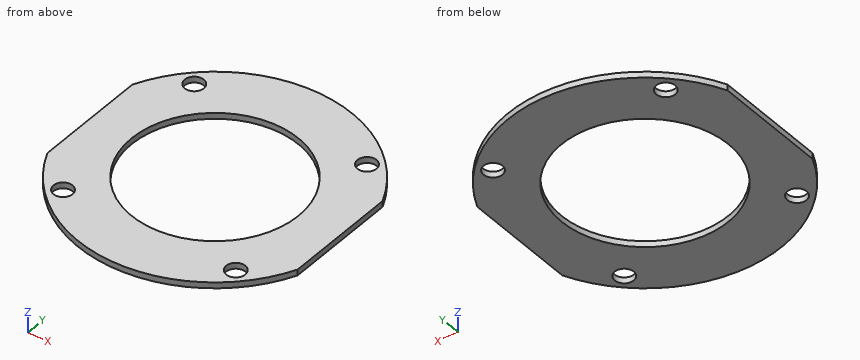
Autodesk Inventor part; units mm, degrees
ref_plane "Work Plane1" through (22, -12.0416, 0) normal (1, 0, 0) x (0, 0, -1)
ref_plane "YZ Plane" through (0, 0, 0) normal (1, 0, 0) x (0, 1, 0)
ref_plane "XZ Plane" through (0, 0, 0) normal (0, 1, 0) x (-1, 0, 0)
sketch "Sketch1" plane through (0, 0, 0) normal (0, 0, 1) x (1, 0, 0)
  circle A0 centre (0, 0) radius 14
  circle A1 centre (0, 0) radius 23
  dimension "d0" = 28
  dimension "d1" = 46
extrude "Extrusion1" add sketch "Sketch1" along normal blind 10
sketch "Sketch2" plane through (0, 0, 10) normal (0, 0, 1) x (1, 0, 0)
  line L0 (0, 0) -> (23, 0) construction
  circle A0 centre (0, 0) radius 23
  circle A1 centre (0, 0) radius 20.5 construction
  line L1 (0, 0) -> (14.4957, 14.4957) construction
  dimension "d35" = 41
  dimension "d34" = 45
hole "For-m3-screws" at (14.4957, 14.4957, 10) direction (0, 0, -1) diameter 3.2 end through all counterbore diameter 7 counterbore depth 8.5
fillet "Fillet3" radius 0.5 2 edges at (14.3283, 17.9917, 5.75) (17.9917, 14.3283, 5.75)
pattern_circular "Circular Pattern1" count 4 over 360 about axis through (0, 0, 0) along (0, 0, 1) of "For-m3-screws", "Fillet3"
sketch "Sketch3" plane through (0, 0, 0) normal (0, 1, 0) x (-1, 0, 0)
  line L0 (23, 3.8135) -> (-23, 1)
  line L1 (-23, 1) -> (-23, 11)
  line L2 (23, 10) -> (-27, 10)
  line L3 (-23, 11) -> (23, 11)
  line L4 (23, 11) -> (23, 3.8135)
  line L5 (-23, 0) -> (-23, 10)
  line L6 (23, 0) -> (23, 10)
  line L7 (-14, 0) -> (14, 0)
  line L8 (-27, 10) -> (-23, 10)
  point P0 (0, 0)
  point P1 (-14.3283, 10)
  point P2 (0, 11)
  point P3 (-17.9917, 10)
  dimension "d14" = 3.5
  dimension "d15" = 1
  dimension "d16" = 1
extrude "Angled-cut" [suppressed]
sketch "Sketch6" plane through (0, 0, 0) normal (0, 1, 0) x (-1, 0, 0)
  line L0 (23, 10) -> (-23, 10)
  line L1 (-23, 10) -> (-23, 1)
  line L2 (-23, 1) -> (23, 1)
  line L3 (23, 1) -> (23, 10)
  line L4 (23, 0) -> (-23, 0)
  line L5 (23, 0) -> (23, 10)
  line L6 (-23, 0) -> (-23, 10)
  point P0 (0, 0)
  point P1 (0, 10)
  dimension "d27" = 1
extrude "Straight-cut" cut sketch "Sketch6" along normal through all both and the other way through all contours L3 L2 L1 L0
sketch "Sketch4" plane through (0, 0, 0) normal (0, 0, 1) x (1, 0, 0)
  line L0 (21, 30) -> (26, 30)
  line L1 (26, 30) -> (26, -30)
  line L2 (26, -30) -> (21, -30)
  line L3 (21, -30) -> (21, 30)
  point P0 (0, 0)
  point P1 (26, 0)
  dimension "d19" = 21
  dimension "d20" = 60
  dimension "d21" = 5
extrude "Extrusion3" cut sketch "Sketch4" along normal blind 10
mirror "Mirror1" about plane through (0, 0, 0) normal (1, 0, 0) of "Extrusion3"
ref_plane "Work Plane1" through (22, -12.0416, 0) normal (1, 0, 0) x (0, 0, -1)
sketch "Sketch8" plane through (22, -12.0416, 0) normal (1, 0, 0) x (0, 0, -1)
  line L0 (-0.5, 21.0416) -> (-0.5, 3.0416) construction
  line L1 (-1, 2.6608) -> (-1, 21.4224)
  line L2 (0, 21.4224) -> (0, 2.6608)
  line L3 (0, 12.0416) -> (-1, 12.0416) construction
  point P0 (-0.5, 12.0416)
  dimension "d41" = 18
hole "Hole2" [suppressed]
chamfer "Chamfer1" [suppressed]
thread "Thread2"
thread "Thread3"
thread "Thread4"
thread "Thread5"
equation "\"d0\" = innerdiameter"
equation "\"d1\" = outerdiameter"
equation "\"d35\" = holepositiondiameter"
equation "\"outerdiameter\" = 46"
equation "\"innerdiameter\" = 28"
equation "\"holepositiondiameter\" = 41"
equation "\"trimspan\" = 21"
properties part number "probe-gate-spacer-quartz-holder" material "Stainless Steel"
The listing builds one solid part. Answer for the finished solid, in the listing's coordinates (mm). Round coordinates to 2 decimals unless told otherwise and drop trailing zeros. Loops run counter-clockwise (first coordinate to the right, second up) from the corner with the lowest first, then second, coordinate; pieces in that order, holes last.
1) A cutting plane is placed at D-D on y = -15. Determine the outline of the cut face in (x, z), plus the area to 3 significant figures.
Outcome:
outline: (-17.44, 0) - (-16.01, 0) - (-16.01, 1) - (-17.44, 1) - close; (-12.98, 0) - (12.98, 0) - (12.98, 1) - (-12.98, 1) - close; (16.01, 0) - (17.44, 0) - (17.44, 1) - (16.01, 1) - close
area: 28.8 mm2
2) Consider line 1 (Y direction, x = 0, z = 0.7); line 2 (X direction, y = -15, z = 0.8); line 3 (X direction, y = 0, z = 0.55). Determine where each line is inside the solid, lowest interval first.
Outcome:
line 1: y = -23 to -14, 14 to 23
line 2: x = -17.44 to -16.01, -12.98 to 12.98, 16.01 to 17.44
line 3: x = -21 to -14, 14 to 21
3) A cutting plane is placed at B-B on x = 0. Determine the outline of the cut face in (y, z), plus the area to 3 significant figures.
Outcome:
outline: (-23, 0) - (-14, 0) - (-14, 1) - (-23, 1) - close; (14, 0) - (23, 0) - (23, 1) - (14, 1) - close
area: 18.0 mm2
4) A cutting plane is placed at A-A on y = 0. Determine the outline of the cut face in (x, z).
Outcome:
outline: (-21, 0) - (-14, 0) - (-14, 1) - (-21, 1) - close; (14, 0) - (21, 0) - (21, 1) - (14, 1) - close
5) A cutting plane is placed at C-C on x = -13.5. Determine the outline of the cut face in (y, z).
Outcome:
outline: (-18.62, 0) - (-15.75, 0) - (-15.75, 1) - (-18.62, 1) - close; (-13.24, 0) - (-3.71, 0) - (-3.71, 1) - (-13.24, 1) - close; (3.71, 0) - (13.24, 0) - (13.24, 1) - (3.71, 1) - close; (15.75, 0) - (18.62, 0) - (18.62, 1) - (15.75, 1) - close
